Source: CAD feature listing. Evaluate the final solid. Frame: model axes, mm. A direction names the side the tool comes from. Coordinates: 2 decimals unless noted, no trailing zeros. Order: outer loops, then holes, each group sorted by start corner. A loop starts at its lowest first (then second) coordinate and runs counter-clockwise, first axis right, second up. Notation, with made-up numbers: (-30.75, -13) -> (21.25, -13) arc R32 cw to (21.25, 26) -> close; hole circle Ø1 at (60, 42). An arc over 180 degrees is marked (long way). Put each result on its own line as item: value.
from build123d import *

# Parameters (mm, degrees)
F1_DEPTH  = 15.05
F3_DEPTH  = 7.6
F5_R      = 11
F5_R_2    = 5
F6_DEPTH  = 2.9
F5_R_3    = 2.5
F7_DEPTH  = 23.25
F9_DEPTH  = 15.4
F10_W     = 16
F10_H     = 7.6
F11_DEPTH = 6.45
F5_R_4    = 1.25
F12_DEPTH = 3.75


with BuildPart() as f1:
    # F0 (on Top) → F1 (new body, symmetric)
    with BuildSketch(Plane.XY):
        Polygon((21.125, 14.2244820946), (14.6871989155, 21.125), (-14.6871989155, 21.125), (-21.125, 14.2244820946), (-21.125, -14.2244820946), (-14.6871989155, -21.125), (14.6871989155, -21.125), (21.125, -14.2244820946), align=None)
    extrude(amount=F1_DEPTH, both=True)

    # F2 (on face) → F3 (join)
    with BuildSketch(Plane.XY.offset(15.05)):
        Polygon((-21.2083792326, 16.6279797649), (-21.125, 14.2244820946), (-21.125, -14.2244820946), (-21.125, -16.7187881371), (-17.2214704386, -21.125), (-14.6871989155, -21.125), (14.6871989155, -21.125), (17.2214704386, -21.125), (21.125, -16.7187881371), (21.125, -14.2244820946), (21.125, 14.2244820946), (21.2083792326, 16.6279797649), (17.3048496711, 21.0341916278), (14.6871989155, 21.125), (-14.6871989155, 21.125), (-17.3048496711, 21.0341916278), align=None)
    extrude(amount=F3_DEPTH)

    # F4: F1 across plane


with BuildPart() as f1_1:
    add(f1.part)
    add(f1.part.mirror(Plane.XY))

    # F5 (on face) → F6 (join)
    with BuildSketch(Plane.XY.offset(22.65)):
        Circle(F5_R)
        Circle(F5_R_2, mode=Mode.SUBTRACT)
    extrude(amount=F6_DEPTH)

    # F5 (on face) → F7 (join)
    with BuildSketch(Plane.XY.offset(22.65)):
        Circle(F5_R_3)
    extrude(amount=F7_DEPTH)

    # F8 (on face) → F9 (cut)
    with BuildSketch(Plane.XY.offset(45.9)):
        with BuildLine():
            ThreePointArc((-2, 1.5), (-2.5, 0), (-2, -1.5))
            Line((-2, -1.5), (-2, 1.5))
        make_face()
    extrude(amount=-F9_DEPTH, mode=Mode.SUBTRACT)

    # F10 (on face) → F11 (join)
    with BuildSketch(Plane.YZ.offset(21.125)):
        with Locations((0, -18.85)):
            Rectangle(F10_W, F10_H)
    extrude(amount=F11_DEPTH)

    # F5 (on face) → F12 (cut)
    with BuildSketch(Plane.XY.offset(22.65)):
        with Locations((-15.5, -15.5)):
            Circle(F5_R_4)
        with Locations((15.5, -15.5)):
            Circle(F5_R_4)
        with Locations((15.5, 15.5)):
            Circle(F5_R_4)
        with Locations((-15.5, 15.5)):
            Circle(F5_R_4)
    extrude(amount=-F12_DEPTH, mode=Mode.SUBTRACT)


solid = f1_1.part
1. Cut plane B-B on z = 3. Output: boundary loops of the cut face in (x, y) (3 decimals).
Numbers:
outline: (-21.125, -14.224) -> (-14.687, -21.125) -> (14.687, -21.125) -> (21.125, -14.224) -> (21.125, 14.224) -> (14.687, 21.125) -> (-14.687, 21.125) -> (-21.125, 14.224) -> close
2. Pull-direction query (Z, two-part tool) for faces 1 (the flat face through (2, -5, 25.55)), 2 (the cylindrical face through (-15.66, -14.26, 20.8)), 3 (the flat face through (17.861, -17.723, 0.211)); classes: pulls with the +Z half, pulls with the -Z half, needs draft (parallel to the pull), parting line crosses it, or undercut.
Numbers:
face 1: pulls with the +Z half
face 2: needs draft
face 3: undercut
3. Ray query, line 1 along Y through (x, z) = (0, 24); line 2 along Y through (x, z) = (-15.5, 21.3) (3 decimals); line 3 along X through (y, z) = (6.5, 21.5) (3 decimals). Return the intervals inside material, ascending.
Numbers:
line 1: y = -11 to -5, -2.5 to 2.5, 5 to 11
line 2: y = -21.125 to -16.75, -14.25 to 14.25, 16.75 to 21.097
line 3: x = -21.125 to 21.125
4. Set-up query: faces 4 (the cylindrical face through (15.34, -14.26, 20.8)), 5 (the flat face through (24, 0, -15.05)), 6 (the flat face through (-2, 0, 38)). Return all of +Z, -Z, +X, -X, +Y, -Y with unobstructed straight access to the full face (end or side cutting, diameter ignored); none if empty.
Numbers:
face 4: +Z
face 5: +Z, +X, +Y, -Y
face 6: +Z, -X, +Y, -Y
5. Cut plane D-D on z = 17. Output: boundary loops of the cut face in (x, y) (3 decimals), plus the area to 3 significant figures.
Numbers:
outline: (-21.208, 16.628) -> (-21.125, 14.224) -> (-21.125, -16.719) -> (-17.221, -21.125) -> (17.221, -21.125) -> (21.125, -16.719) -> (21.125, 14.224) -> (21.208, 16.628) -> (17.305, 21.034) -> (14.687, 21.125) -> (-14.687, 21.125) -> (-17.305, 21.034) -> close
area: 1,750 mm2
6. Cut plane C-C on x = 22. Output: boundary loops of the cut face in (y, z).
Numbers:
outline: (-8, -22.65) -> (8, -22.65) -> (8, -15.05) -> (-8, -15.05) -> close
7. Cut plane A-A on y = 0. Output: boundary loops of the cut face in (x, z) (3 decimals), plus the area to 3 significant figures.
Numbers:
outline: (-21.125, -22.65) -> (27.575, -22.65) -> (27.575, -15.05) -> (21.125, -15.05) -> (21.125, 22.65) -> (11, 22.65) -> (11, 25.55) -> (5, 25.55) -> (5, 22.65) -> (2.5, 22.65) -> (2.5, 45.9) -> (-2, 45.9) -> (-2, 30.5) -> (-2.5, 30.5) -> (-2.5, 22.65) -> (-5, 22.65) -> (-5, 25.55) -> (-11, 25.55) -> (-11, 22.65) -> (-21.125, 22.65) -> close
area: 2,110 mm2
8. First-contact query: pin 1 (24 mm diameter, centred on x = 0.5, y = 5, fed in from +Z); pin 2 (2 mm diameter, centred on x = 15.5, y = -16, fed in from +Z); pin 3 (10 mm diameter, centred on y = 14.5, z = 11, fed in from +X); pin 4 (10 mm diameter, centred on x = -10, y = -5, fed in from +Z). Flat tips, straight axial feed; report the tip coordinate or a pass-through.
Numbers:
pin 1: stops at z = 45.9
pin 2: stops at z = 22.65
pin 3: stops at x = 21.21
pin 4: stops at z = 25.55
